```python
from build123d import *

# Parameters (mm, degrees)
SKETCH1_W           = 50.8
SKETCH1_H           = 76.2
SKETCH1_R           = 2.54
BOSS_EXTRUDE1_DEPTH = 5.08
SKETCH2_R           = 2.1
CUT_EXTRUDE1_DEPTH  = 4


with BuildPart() as part:
    # Sketch1 → Boss-Extrude1 (new body)
    with BuildSketch(Plane.XY):
        with Locations((-23.244105975, 56.042212855)):
            Rectangle(SKETCH1_W, SKETCH1_H)
        with Locations((-38.484105975, 25.562212855)):
            Circle(SKETCH1_R, mode=Mode.SUBTRACT)
        with Locations(Location((-8.004105975, 25.562212855, 0), (0, 0, 180))):
            Circle(SKETCH1_R, mode=Mode.SUBTRACT)
        with Locations((-8.004105975, 86.522212855)):
            Circle(SKETCH1_R, mode=Mode.SUBTRACT)
        with Locations(Location((-38.484105975, 86.522212855, 0), (0, 0, 180))):
            Circle(SKETCH1_R, mode=Mode.SUBTRACT)
    extrude(amount=BOSS_EXTRUDE1_DEPTH)

    # Sketch2 → Cut-Extrude1 (cut)
    with BuildSketch(Plane.XZ.offset(-17.942212855)):
        with Locations(Location((-38.438159235, 2.54, 0), (0, 0, 270))):
            Circle(SKETCH2_R)
        with Locations(Location((-8.050052715, 2.54, 0), (0, 0, 90))):
            Circle(SKETCH2_R)
    extrude(amount=-CUT_EXTRUDE1_DEPTH, mode=Mode.SUBTRACT)


solid = part.part
```
Can you work these out from the model? Positions are in its coordinate system, mm. A direction names the side the tool comes from. Round coordinates to 2 decimals unless told otherwise and drop trailing zeros. Loops run counter-clockwise (first coordinate to the right, second up) from the corner with the lowest first, then second, coordinate; pieces in that order, holes last.
Item 1: Suppose I cut it at A-A, the plane z = 2.6. Write out the boundary of the cut face in (x, y).
Item 2: Which directions (+Z, -Z, +X, -X, +Y, -Y) give clear straight access to the entire face, cutting with the end or side of a thin tool? Please do faces 4 (the cylindrical face through (-10.132, 19.914, 2.267)), 5 (the flat face through (-24, 17.942, 3)).
Item 3: Please list where these lines run through material, in increasing order: L1, parallel to X at y = 87, z = 4; L2, parallel to X at y = 24.5, z = 3.7; L3, parallel to Y at x = -9, z = 4.85.
Item 4: If we mould it in two halves opening along X, with no side actions, what happens to faces 1 (the cylindrical face through (-7.45, 28.04, 2.5)), 2 (the flat face through (-24, 94.142, 3)), 3 (the flat face through (2.156, 56, 3))? For each: +X half, -X half, draft (parallel to the pull), parting line (faces both ways), or undercut.
Item 5: Will these pins go through, and if not, where does the flat tip stop? pin 1 Ø8 at (x, y) = (-38.48, 25.56) entering from +Z; pin 2 Ø3 at (x, y) = (-8, 86.52) entering from -Z.
Reported:
1. outline: (-48.64, 17.94) - (-40.54, 17.94) - (-40.54, 21.94) - (-36.34, 21.94) - (-36.34, 17.94) - (-10.15, 17.94) - (-10.15, 21.94) - (-5.95, 21.94) - (-5.95, 17.94) - (2.16, 17.94) - (2.16, 94.14) - (-48.64, 94.14) - close; hole circle Ø5.08 at (-38.48, 25.56); hole circle Ø5.08 at (-38.48, 86.52); hole circle Ø5.08 at (-8, 25.56); hole circle Ø5.08 at (-8, 86.52)
2. face 4: -Y
2. face 5: +Z, -Z, +X, -X, -Y
3. L1: x = -48.64 to -40.98, -35.99 to -10.5, -5.51 to 2.16
3. L2: x = -48.64 to -40.79, -36.18 to -10.31, -5.7 to 2.16
3. L3: y = 17.94 to 23.23, 27.9 to 84.19, 88.86 to 94.14
4. face 1: undercut
4. face 2: draft
4. face 3: +X half
5. pin 1: stops at z = 5.08
5. pin 2: passes through
